The model under review builds one solid part; all positions refer to its coordinate system, in mm. Round coordinates to 2 decimals unless told otherwise and drop trailing zeros. Loops run counter-clockwise (first coordinate to the right, second up) from the corner with the lowest first, then second, coordinate; pieces in that order, holes last. Notation, with made-up numbers: M -12.5,82.5 L 24.5,82.5 A30 cw 24.5,115.5 Z; hole C 9,61.25 d8. An arc over 180 degrees is marked long. One line per question, with ' | ' between items.
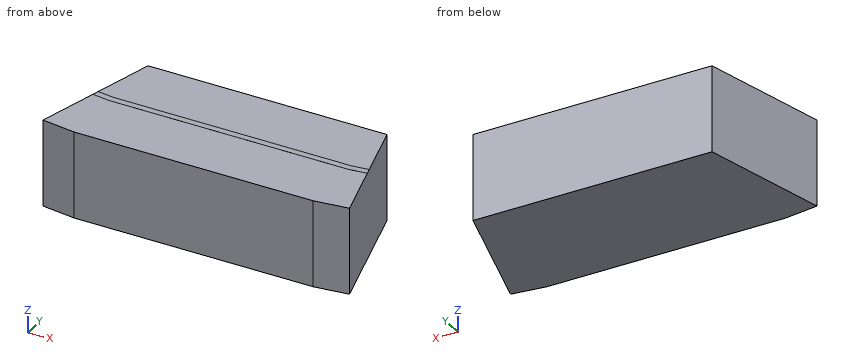
Autodesk Inventor part; units mm, degrees
ref_plane "YZ Plane" through (0, 0, 0) normal (1, 0, 0) x (0, 1, 0)
ref_plane "XZ Plane" through (0, 0, 0) normal (0, 1, 0) x (-1, 0, 0)
ref_plane "XY Plane" through (0, 0, 0) normal (0, 0, 1) x (1, 0, 0)
sketch "スケッチ1" plane through (0, 0, 0) normal (0, 0, 1) x (1, 0, 0)
  line L0 (-550, 300) -> (550, 300)
  line L1 (550, 300) -> (550, -300)
  line L2 (550, -300) -> (-550, -300)
  line L3 (-550, -300) -> (-550, 300)
  line L4 (-550, 300) -> (-705.2914, -279.5555)
  line L5 (-705.2914, -279.5555) -> (-550, -300)
  line L6 (-550, 0) -> (-627.6457, 10.2223)
  line L7 (550, 300) -> (705.2914, -279.5555)
  line L8 (705.2914, -279.5555) -> (550, -300)
  point P0 (0, 0)
  point P1 (0, 300)
  point P2 (550, 0)
  dimension "d0" = 600
  dimension "d1" = 1100
  dimension "d2" = 15
  dimension "d3" = 600
  dimension "d4" = 600
  dimension "d5" = 15
extrude "押し出し1" add sketch "スケッチ1" along normal blind 400
sketch "スケッチ2" plane through (0, 0, 400) normal (0, 0, 1) x (1, 0, 0)
  line L0 (-550, 300) -> (-705.2914, -279.5555)
  line L1 (705.2914, -279.5555) -> (550, 300)
  line L2 (550, 300) -> (-550, 300)
  line L3 (-550, 300) -> (-550, -300)
  line L4 (550, -300) -> (550, 300)
  line L5 (-627.6457, 10.2223) -> (-550, 0)
  line L6 (550, 0) -> (-550, 0)
  line L7 (550, 0) -> (627.6457, 10.2223)
  line L8 (-631.5615, -4.3917) -> (-550.9832, -15)
  line L9 (-550.9832, -15) -> (550.9832, -15)
  line L10 (550.9832, -15) -> (631.5615, -4.3917)
  line L11 (-623.7299, 24.8362) -> (-549.0168, 15)
  line L12 (-549.0168, 15) -> (549.0168, 15)
  line L13 (549.0168, 15) -> (623.7299, 24.8362)
  line L14 (631.5615, -4.3917) -> (623.7299, 24.8362)
  line L15 (-631.5615, -4.3917) -> (-623.7299, 24.8362)
  point P0 (0, 0)
  dimension "d8" = 15
  dimension "d10" = 15
  dimension "d11" = 30
  dimension "d12" = 15
  dimension "d13" = 30
  dimension "d14" = 15
extrude "押し出し2" add sketch "スケッチ2" along normal blind 0.1 contours L11 L3 L5 L0 | L11 L12 L13 L4 L6 L3 | L5 L3 L9 L8 L0 | L1 L7 L4 L13 | L6 L4 L9 L3 | L1 L10 L9 L4 L7
properties part number "Hill 2"
1) Insertion check: P1, Ø2, axis at x = -557.5, y = 123.5, coming from the +Z side; P2, Ø1.5, axis at x = -523.5, y = 162, coming from the -Z side; P3, Ø6, axis at y = -5.5, z = 341.5, coming from the -X side; P4, Ø1.5, axis at y = -163, z = 308, coming from the +X side. Each pin has a flat end and moves straight along its axis. Give the tip position at first contact, or say it passes through.
Output values:
P1: stops at z = 400 | P2: stops at z = 0 | P3: stops at x = -632.66 | P4: stops at x = 674.26
2) Add section D-D on y = -46.5. State the section outline as (x, z) points.
Output values:
outline: M -642.84,0 L 642.84,0 L 642.84,400 L -642.84,400 Z
3) Add section C-C on y = 199.5. State the section outline as (x, z) points, then the cut area to 3 significant figures.
Output values:
outline: M -576.93,0 L 576.93,0 L 576.93,400 L -576.93,400 Z | area: 462,000 mm²
4) For line 1 (Z direction, x = -456.5, y = -34); line 2 (X direction, y = 240.5, z = 19); line 3 (X direction, y = 238.5, z = 147.5), list the stretches that pass through material, from the lowest coordinate up.
Output values:
line 1: z = 0 to 400 | line 2: x = -565.94 to 565.94 | line 3: x = -566.48 to 566.48
5) Add section A-A on z = 264. State the section outline as (x, y) points, then the cut area to 3 significant figures.
Output values:
outline: M -705.29,-279.56 L -550,-300 L 550,-300 L 705.29,-279.56 L 550,300 L -550,300 Z | area: 753,000 mm²
6) Add section B-B on x = -582. State the section outline as (y, z) points.
Output values:
outline: M -295.79,0 L 180.57,0 L 180.57,400 L 19.34,400 L 19.34,400.1 L -10.92,400.1 L -10.92,400 L -295.79,400 Z
